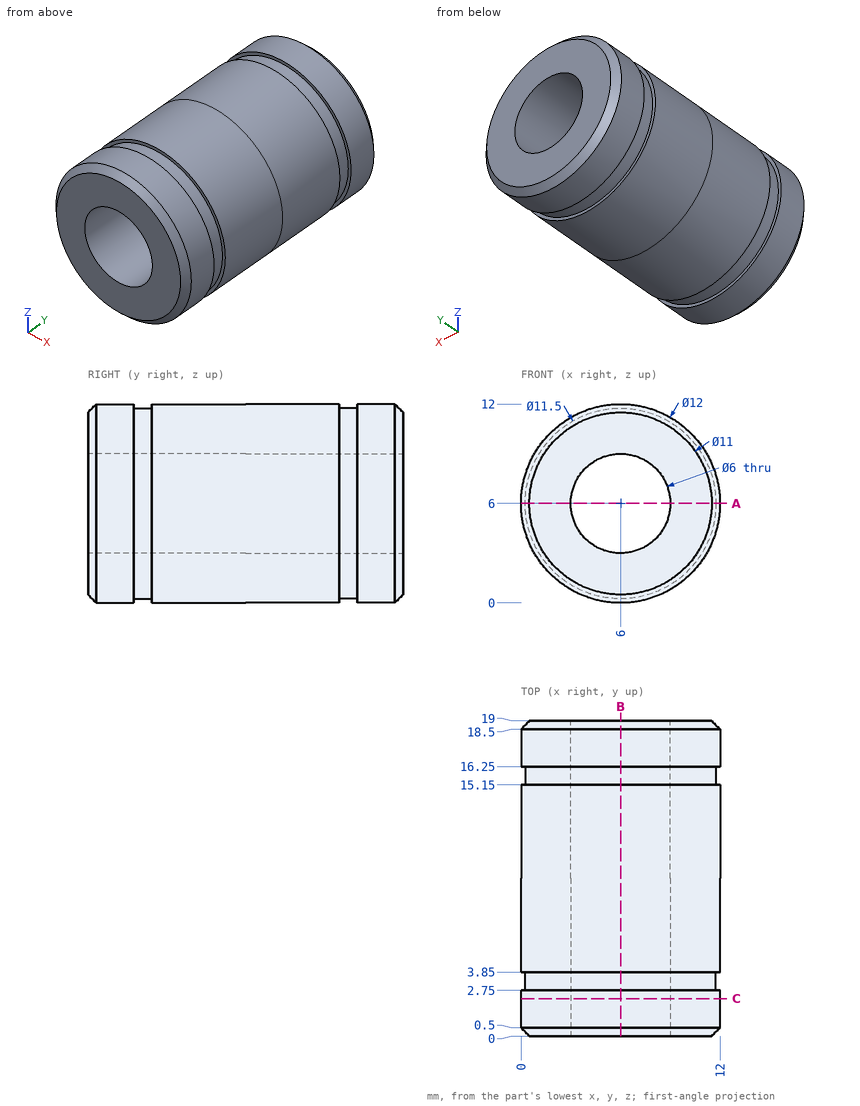
Check sheet for the drawn part. Datum: minimum x, y, z corner. Units: mm. Round coordinates to 2 decimals unless told otherwise and drop trailing zeros. Write each loop counter-clockwise with the first axis right and the second up, starting at its lowest first coordinate (ties: lowest second). Pieces come first, ordered by that corner, then holes. Notation, with made-up numbers: (62, 37.25) - (108, 37.25) arc R16 ccw to (108, 68.25) - close; hole circle Ø8 at (29, 2). An arc over 180 degrees is marked (long way). Return JSON: item names as keys, results as strings.
Q1. Cross-section at B-B (x = 6). Record the boundary of the cut face in (y, z), then the cut area to 3 significant figures.
Returned:
{"outline": "(0, 0.5) - (0.5, 0) - (2.75, 0) - (2.75, 0.25) - (3.85, 0.25) - (3.85, 0) - (15.15, 0) - (15.15, 0.25) - (16.25, 0.25) - (16.25, 0) - (18.5, 0) - (19, 0.5) - (19, 3) - (0, 3) - close; (0, 9) - (19, 9) - (19, 11.5) - (18.5, 12) - (16.25, 12) - (16.25, 11.75) - (15.15, 11.75) - (15.15, 12) - (3.85, 12) - (3.85, 11.75) - (2.75, 11.75) - (2.75, 12) - (0.5, 12) - (0, 11.5) - close", "area": "112 mm²"}
Q2. Scan lines: L1, parallel to X at y = 17, z = 6; L2, parallel to Z at x = 5.25, y = 2.5. Record each from-to range of solid material in increasing order. Write a range as from..to.
Returned:
{"L1": "x = 0..3, 9..12", "L2": "z = 0.05..3.1, 8.9..11.95"}
Q3. Cross-section at A-A (z = 6). Record the boundary of the cut face in (x, y).
Returned:
{"outline": "(0, 0.5) - (0.5, 0) - (3, 0) - (3, 19) - (0.5, 19) - (0, 18.5) - (0, 16.25) - (0.25, 16.25) - (0.25, 15.15) - (0, 15.15) - (0, 3.85) - (0.25, 3.85) - (0.25, 2.75) - (0, 2.75) - close; (9, 0) - (11.5, 0) - (12, 0.5) - (12, 2.75) - (11.75, 2.75) - (11.75, 3.85) - (12, 3.85) - (12, 15.15) - (11.75, 15.15) - (11.75, 16.25) - (12, 16.25) - (12, 18.5) - (11.5, 19) - (9, 19) - close"}
Q4. Depth check by flat-ended pin: P1, Ø2, axis at x = 3, y = 12.5, coming from the -Z side; P2, Ø4, axis at y = 11, z = 3.5, coming from the +X side; P3, Ø4, axis at y = 16.5, z = 2.5, coming from the +X side. Enter the tip coordinate at first touch or a pass-through.
Returned:
{"P1": "stops at z = 0.34", "P2": "stops at x = 11.98", "P3": "stops at x = 11.81"}
Q5. Cross-section at C-C (y = 2.25). Record the boundary of the cut face in (x, z).
Returned:
{"outline": "circle Ø12 at (6, 6); hole circle Ø6 at (6, 6)"}
